The model under review builds one solid part; all positions refer to its coordinate system, in mm. Face numbers are marked on the shaded views. A direction names the side the tool comes from. Give positions to 0.01 mm unless a question says otherwise; leave off trailing zeros. Write each loop counter-clockwise with the first axis right and the second up, starting at its lowest first coordinate (ties: lowest second). Pieces come first, ordered by that corner, then holes. Notation, with made-up numbers: (51.25, 60) - (84.25, 60) arc R13 ccw to (84.25, 69) - close; hole circle Ø3 at (57, -23.75). An arc over 180 degrees is marked (long way). One line per question, with ' | ' between items. Start each with the question number.
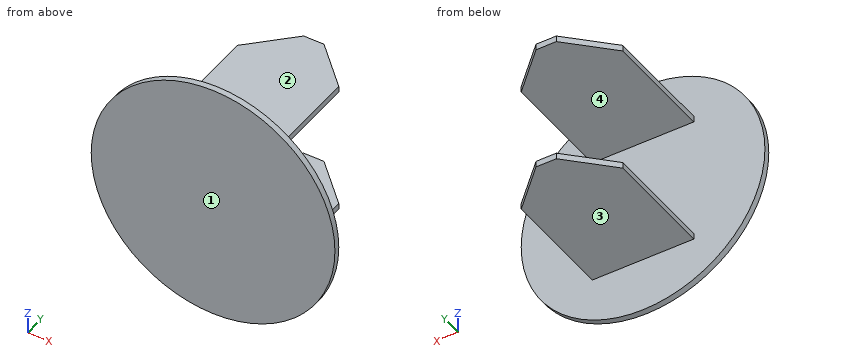
Autodesk Inventor part; units mm, degrees
ref_plane "YZ Plane" through (0, 0, 0) normal (1, 0, 0) x (0, 1, 0)
ref_plane "XZ Plane" through (0, 0, 0) normal (0, 1, 0) x (-1, 0, 0)
ref_plane "XY Plane" through (0, 0, 0) normal (0, 0, 1) x (1, 0, 0)
sketch "Esquisse1" plane through (0, 0, 0) normal (0, 1, 0) x (-1, 0, 0)
  circle A0 centre (0, 0) radius 60
  dimension "d0" = 120
extrude "Extrusion1" add sketch "Esquisse1" along normal blind 3
sketch "Esquisse2" plane through (0, 3, 0) normal (0, 1, 0) x (1, 0, 0)
  line L0 (-25, -33) -> (25, -33)
  line L1 (25, -33) -> (25, -30)
  line L2 (25, -30) -> (-25, -30)
  line L3 (-25, -30) -> (-25, -33)
  line L4 (-25, 33) -> (25, 33)
  line L5 (25, 33) -> (25, 30)
  line L6 (25, 30) -> (-25, 30)
  line L7 (-25, 30) -> (-25, 33)
  point P0 (0, 0)
  dimension "d3" = 50
  dimension "d4" = 50
  dimension "d5" = 30
  dimension "d7" = 30
  dimension "d8" = 3
  dimension "d9" = 3
  dimension "d10" = 25
extrude "Extrusion2" add sketch "Esquisse2" along normal blind 75
chamfer "Chanfrein1" distance 20 angle 45 4 edges at (25, 78, 31.5) (25, 78, -31.5) (-25, 78, -31.5) (-25, 78, 31.5)
properties part number "Bras principal"
Item 1: Machinability: for the marked faces 1, 2, 3 and 4, which of the approach directions +Z, -Z, +X, -X, +Y, -Y give a long, thin tool a straight path to every point of the face, cutting with its end or side? Answer none if there is none.
Item 2: Take a section at A-A (y = 5.5). Give the boundary of the cut face in (x, z).
Item 3: For probe 1 along Z at (x, y) = (10, 26.5); probe 2 along Y at (x, z) = (-6, -39); probe 3 along X at (y, z) = (33, -32), list the stretches that pass through material, from the lowest coordinate up.
Item 4: Clearance check with flat-ended pins moving along their axes: P1, Ø1.5, axis at x = 13, y = 41.5, coming from the +Z side; P2, Ø12, axis at y = 46, z = -24.5, coming from the +X side; P3, Ø3.5, axis at y = 29.5, z = -32, coming from the -X side. State where each tip first meets the part, or that it passes through.
Item 5: Take a section at B-B (x = 0). Give the boundary of the cut face in (y, z), plus the area to 3 significant figures.
Item 6: Take a section at C-C (z = 0). Give the boundary of the cut face in (x, y).
Item 7: Take a section at D-D (x = -18). Give the boundary of the cut face in (y, z).
Check sheet entries:
1) face 1: +Z, -Z, +X, -X, -Y | face 2: +Z, +X, -X, +Y | face 3: -Z, +X, -X, +Y | face 4: +X, -X, +Y
2) outline: (-25, -33) - (25, -33) - (25, -30) - (-25, -30) - close; (-25, 30) - (25, 30) - (25, 33) - (-25, 33) - close
3) probe 1: z = -33 to -30, 30 to 33 | probe 2: y = 0 to 3 | probe 3: x = -25 to 25
4) P1: stops at z = 33 | P2: stops at x = 25 | P3: stops at x = -25
5) outline: (0, -60) - (3, -60) - (3, -33) - (78, -33) - (78, -30) - (3, -30) - (3, 30) - (78, 30) - (78, 33) - (3, 33) - (3, 60) - (0, 60) - close | area: 810 mm^2
6) outline: (-60, 0) - (60, 0) - (60, 3) - (-60, 3) - close
7) outline: (0, -57.24) - (3, -57.24) - (3, -33) - (65, -33) - (65, -30) - (3, -30) - (3, 30) - (65, 30) - (65, 33) - (3, 33) - (3, 57.24) - (0, 57.24) - close
